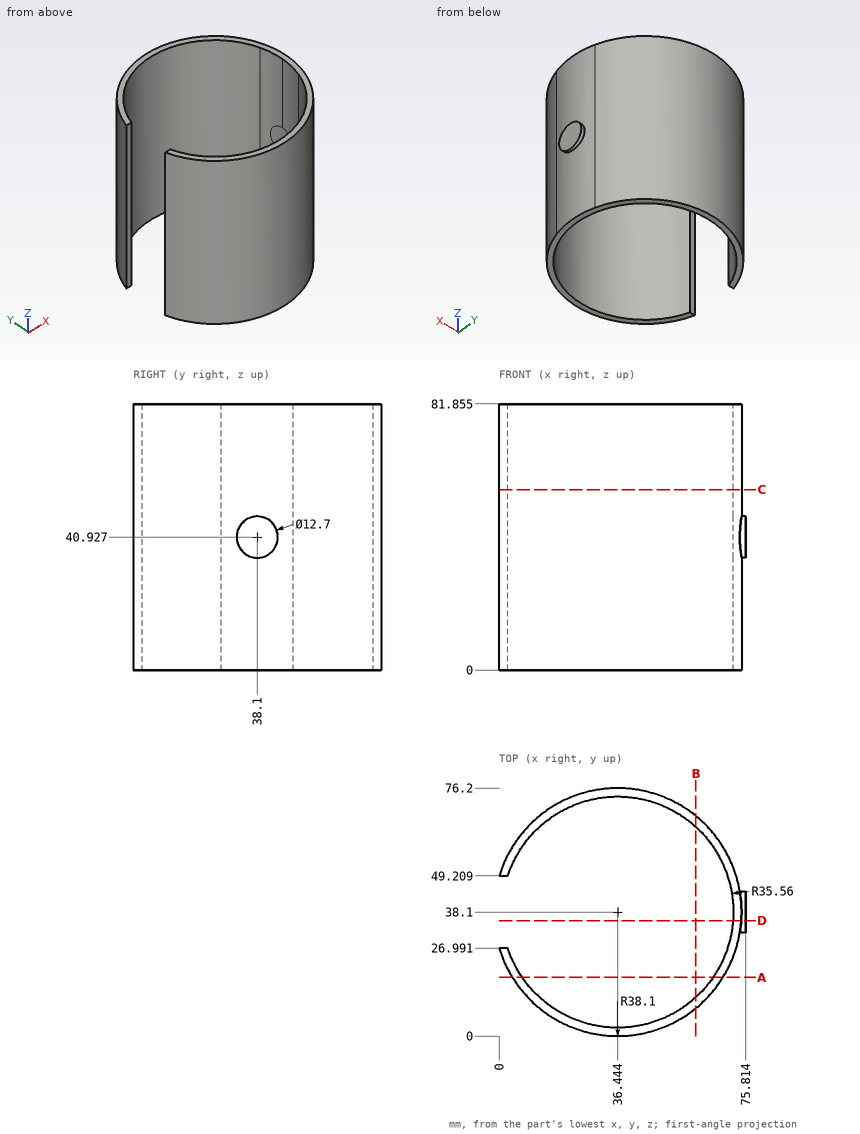
For this review, use the dimensioned drawing (mm, ordinates from the lowest corner) and the shaded views. Round coordinates to 2 decimals unless told otherwise and drop trailing zeros. Write each loop counter-clockwise with the first axis right and the second up, starting at its lowest first coordinate (ties: lowest second). Pieces come first, ordered by that corner, then holes. Notation, with made-up numbers: (66.5, 75) -> (115.5, 75) arc R6 ccw to (115.5, 86) -> close; hole circle Ø11 at (76, 11). An arc over 180 degrees is marked (long way). Answer in a Markdown table with one row per item.
Q1. To check wall thickness, follow L1, parallel to X at y = 18.5, z = 55 (1 decimal); L2, parallel to X at y = 39, z = 16; L3, parallel to Y at x = 44, z = 26. State the ranges of each line that lie inside material, in increasing order. Write a range as [from, to].
The answers:
| item | result |
|---|---|
| L1 | [3.8, 6.8], [66.1, 69.1] |
| L2 | [71.99, 74.53] |
| L3 | [0.76, 3.35], [72.85, 75.44] |
Q2. Take a section at B-B, the plane x = 60.5. State the section outline as (y, z) points (1 decimal).
The answers:
| item | result |
|---|---|
| outline | (8.6, 0) -> (11.9, 0) -> (11.9, 81.9) -> (8.6, 81.9) -> close; (64.3, 0) -> (67.6, 0) -> (67.6, 81.9) -> (64.3, 81.9) -> close |
Q3. Take a section at C-C, the plane z = 55.5. State the section outline as (x, y) points (1 decimal).
The answers:
| item | result |
|---|---|
| outline | (0, 27) arc R38.1 ccw (long way) to (0, 49.2) -> (2.7, 49.2) arc R35.6 cw (long way) to (2.7, 27) -> close |
Q4. Take a section at A-A, the plane y = 18. State the section outline as (x, z) points (1 decimal).
The answers:
| item | result |
|---|---|
| outline | (4.1, 0) -> (7.1, 0) -> (7.1, 81.9) -> (4.1, 81.9) -> close; (65.8, 0) -> (68.8, 0) -> (68.8, 81.9) -> (65.8, 81.9) -> close |
Q5. Clearance check with flat-ended pins moving along their axes: pin 1 Ø2 at (x, z) = (1.5, 47.5) entering from +Y (1 decimal); pin 2 Ø4 at (y, z) = (20, 61) entering from +X (1 decimal); pin 3 Ø0.8 at (x, z) = (2, 49) entering from -Y (1 decimal). State where each tip first meets the part, or that it passes through.
The answers:
| item | result |
|---|---|
| pin 1 | y = 55.4 |
| pin 2 | x = 71 |
| pin 3 | y = 21 |
Q6. Take a section at D-D, the plane y = 35.5. State the section outline as (x, z) points (1 decimal).
The answers:
| item | result |
|---|---|
| outline | (71.9, 0) -> (74.5, 0) -> (74.5, 35.1) -> (75.8, 35.1) -> (75.8, 46.7) -> (74.5, 46.7) -> (74.5, 81.9) -> (71.9, 81.9) -> close |
